```python
from build123d import *

# Parameters (mm, degrees)
SKETCH2_W           = 60
SKETCH2_H           = 3
SKETCH2_H_2         = 11
BOSS_EXTRUDE2_DEPTH = 2
SKETCH3_W           = 60
SKETCH3_H           = 3
BOSS_EXTRUDE3_DEPTH = 10
SKETCH4_W           = 10
SKETCH4_H           = 2
BOSS_EXTRUDE4_DEPTH = 1
FILLET1_START       = -61
FILLET1_DEPTH       = 62
FILLET2_R           = 1


with BuildPart() as part:
    # Sketch2 → Boss-Extrude2 (new body)
    with BuildSketch(Plane(origin=(0, 0, 0), x_dir=(1, 0, 0), z_dir=(0, 1, 0))):
        with Locations((-30, 1.5)):
            Rectangle(SKETCH2_W, SKETCH2_H)
        with Locations((-30, -5.5)):
            Rectangle(SKETCH2_W, SKETCH2_H_2)
        with Locations((-30, -12.5)):
            Rectangle(SKETCH2_W, SKETCH2_H)
    extrude(amount=BOSS_EXTRUDE2_DEPTH)

    # Sketch3 → Boss-Extrude3 (add)
    with BuildSketch(Plane(origin=(0, 2, 0), x_dir=(1, 0, 0), z_dir=(0, 1, 0))):
        with Locations((-30, -12.5)):
            Rectangle(SKETCH3_W, SKETCH3_H)
        with Locations((-30, 1.5)):
            Rectangle(SKETCH3_W, SKETCH3_H)
    extrude(amount=BOSS_EXTRUDE3_DEPTH)

    # Sketch4 → Boss-Extrude4 (add)
    with BuildSketch(Plane(origin=(0, 0, 11), x_dir=(-1, 0, 0), z_dir=(0, 0, -1))):
        with Locations((49, 11)):
            Rectangle(SKETCH4_W, SKETCH4_H)
        with Locations((11, 11)):
            Rectangle(SKETCH4_W, SKETCH4_H)
    extrude(amount=BOSS_EXTRUDE4_DEPTH)

    # Fillet1: read off the stored shape, not the designer's step
    # Fillet1 outline → Fillet1 (cut)
    with BuildSketch(Plane.YZ.offset(FILLET1_START)):
        with BuildLine():
            Line((12, 0), (10, 0))
            ThreePointArc((10, 0), (11.414213562, -0.585786438), (12, -2))
            Line((12, -2), (12, 0))
        make_face()
        with BuildLine():
            ThreePointArc((12, 12), (11.414213562, 10.585786438), (10, 10))
            Line((10, 10), (12, 10))
            Line((12, 10), (12, 12))
        make_face()
    extrude(amount=FILLET1_DEPTH, mode=Mode.SUBTRACT)

    # Fillet2
    fillet2_edges = [part.edges().sort_by_distance(p)[0] for p in [
        (-60, 6, -3),
        (0, 6, -3),
        (0, 6, 14),
        (-60, 6, 14),
        (-60, 2, 5.5),
        (0, 2, 5.5),
        (0, 12, 13),
        (-30, 2, 11),
        (-30, 2, 0),
        (-60, 12, -2.5),
        (-30, 0, -3),
        (0, 0, 5.5),
        (0, 12, -2.5),
        (0, 6, 0),
        (0, 6.866025404, 11),
        (0, 11.931851652, 11.48236191),
        (0, 11.414213562, -0.585786438),
        (-60, 6, 0),
        (-30, 0, 14),
        (-60, 12, 13),
        (-60, 6.866025404, 11),
        (-60, 11.931851652, 11.48236191),
        (-60, 11.414213562, -0.585786438),
        (-60, 0, 5.5),
    ]]
    fillet(fillet2_edges, radius=FILLET2_R - 0.0001)  # a hair under: the kernel refuses the full size


solid = part.part
```
Work out the finished part from the listing and answer in its coordinate system (mm). A direction names the side the tool comes from. Give positions to 0.01 mm unless a question says otherwise; leave off trailing zeros. Loops run counter-clockwise (first coordinate to the right, second up) from the corner with the lowest first, then second, coordinate; pieces in that order, holes last. Notation, with made-up numbers: M 16.5,56 L 38.5,56 A18 cw 38.5,76 Z; hole C -14,35.25 d4. An arc over 180 degrees is marked long. One line per item, written item: value. Start each with the question number.
1. Find section D-D (x = -46.5). Give the vertices of the cut face in (y, z), and give its area (3 significant figures).
2. Determine the mould class of faces 1 (the face through (-59.715, 1.699, 5.563)), 2 (the face through (-0.301, 6.577, -2.715)), 3 (the face through (-59.715, 0.301, 5.605)), 4 (the face through (-48.9, 10, 10.5)) for opening direction Y: released by +Y, released by -Y, zero draft, split by the parting line, or undercut.
3. Find section C-C (x = -39.5). Give the vertices of the cut face in (y, z), and give its area (3 significant figures).
4. Find the intervals of material crossed by probe 1 along Z at (x, y) = (-14.5, 6.25); probe 2 along Y at (x, z) = (-10.5, 2); probe 3 along Z at (x, y) = (-27, 10.5), in increasing order.
5. Each of these flat-tipped pins is pushed along its axis until it touches: P1, Ø0.8, axis at y = 11, z = 10.5, coming from the +X side; P2, Ø4.5, axis at x = -17.5, z = 5.5, coming from the +Y side; P3, Ø0.8, axis at y = 11.5, z = 10.5, coming from the -X side. Where does it stop, or does it pass through?
6. Find section A-A (y = 8.25). Give the vertices of the cut face in (x, z).
7. Which of the six approach directions +Z, -Z, +X, -X, +Y, -Y give full straight-line access (tool end or side, diameter ignored) to faces 5 (the face through (-0.301, 0.285, 5.395)), 6 (the face through (-54, 10.7, 10.6)), 7 (the face through (-30, 6, 14)), 8 (the face through (-29.594, 2.301, 0.285)), 9 (the face through (-0.301, 7.427, 11.285))?
Reported:
1. outline: M 0,-2 A1 ccw 1,-3 L 12,-3 L 12,-2 A2 ccw 10,0 L 3,0 A1 cw 2,1 L 2,10 A1 cw 3,11 L 10,11 L 10,10 A2 ccw 12,12 L 12,14 L 1,14 A1 ccw 0,13 Z
1. area: 94.3 mm²
2. face 1: released by +Y
2. face 2: zero draft
2. face 3: released by -Y
2. face 4: undercut
3. outline: M 0,-2 A1 ccw 1,-3 L 12,-3 L 12,-2 A2 ccw 10,0 L 3,0 A1 cw 2,1 L 2,10 A1 cw 3,11 L 11.73,11 A2 ccw 12,12 L 12,14 L 1,14 A1 ccw 0,13 Z
3. area: 93.1 mm²
4. probe 1: z = -3 to 0, 11 to 14
4. probe 2: y = 0 to 2
4. probe 3: z = -3 to -0.06, 11 to 14
5. P1: stops at x = -6
5. P2: stops at y = 2
5. P3: stops at x = -54
6. outline: M -60,-2 A1 ccw -59,-3 L -1,-3 A1 ccw 0,-2 L 0,-1 A1 ccw -1,0 L -59,0 A1 ccw -60,-1 Z; M -60,12 A1 ccw -59,11 L -1,11 A1 ccw 0,12 L 0,13 A1 ccw -1,14 L -59,14 A1 ccw -60,13 Z
7. face 5: +Z, -Z, +X, -Y
7. face 6: -X, +Y
7. face 7: +Z, +X, -X, +Y, -Y
7. face 8: +X, -X, +Y
7. face 9: +X, +Y
